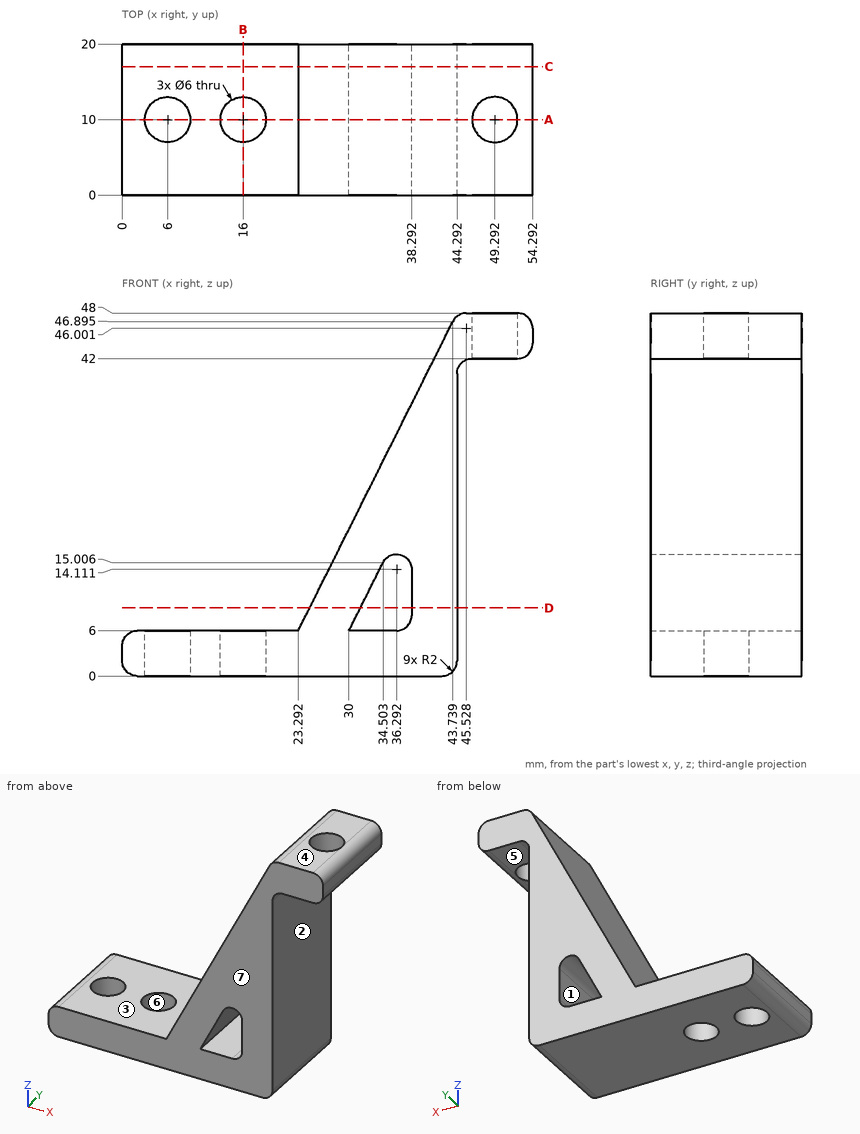
Check sheet for the drawn part. Datum: minimum x, y, z corner. Units: mm. A direction names the side the tool comes from. Round coordinates to 2 decimals unless told otherwise and drop trailing zeros. Loops run counter-clockwise (first coordinate to the right, second up) from the corner with the lowest first, then second, coordinate; pieces in that order, holes last. Notation, with made-up numbers: (80, 10) - (114, 10) arc R13 cw to (114, 29) - close; hole circle Ø8 at (8.25, -23.5). An arc over 180 degrees is marked (long way). Write item = value, one per line. Start each with the question number.
1. Section check D-D on z = 9. Enter the section's corners in (x, y).
2. Depth check by flat-ended pin: pin 1 (5 mm diameter, centred on y = 15, z = 16.5, fed in from -X); pin 2 (3 mm diameter, centred on x = 19.5, y = 10.5, fed in from +Z); pin 3 (7 mm diameter, centred on x = 32.5, y = 10, fed in from +Z) (1 decimal). Enter the tip coordinate at first touch or a pass-through.
3. Set-up check for the marked faces 1, 2, 3 and 4: record each of +Z, -Z, +X, -X, +Y, -Y from which the full face is reachable in a straight line by a thin tool's end or side.
4. Section check C-C on y = 17. Enter the section's corners in (x, z) (1 decimal), then the cut area to 3 significant figures.
5. Thickness scan on line 1 (Y direction, x = 6, z = 2.9); line 2 (X direction, y = 8.75, z = 12.5); line 3 (Z direction, x = 18, y = 7.5). Record the ranges inside material, lowest first.
6. Section check B-B on x = 16. Enter the section's corners in (y, z).
7. Section check A-A on y = 10. Give the number of separate pieces and of enclosed holes in the cut face, then the cut area to 3 significant figures.
8. Mould release check, pull along Y, two halves, no side actions. Record for the marked faces 5, 6 and 7: released by +Y, released by -Y, zero draft, split by the parting line, or undercut.
Working result:
q1.outline = (24.79, 0) - (31.5, 0) - (31.5, 20) - (24.79, 20) - close; (38.29, 0) - (44.29, 0) - (44.29, 20) - (38.29, 20) - close
q2.pin_1 = 27.29
q2.pin_2 = 6
q2.pin_3 = 31.4
q3.face_1 = +Y, -Y
q3.face_2 = -Z, +X, +Y, -Y
q3.face_3 = +Z, -X, +Y, -Y
q3.face_4 = +Z, +X, -X, +Y, -Y
q4.outline = (0, 2) arc R2 ccw to (2, 0) - (42.3, 0) arc R2 ccw to (44.3, 2) - (44.3, 40) arc R2 cw to (46.3, 42) - (52.3, 42) arc R2 ccw to (54.3, 44) - (54.3, 46) arc R2 ccw to (52.3, 48) - (45.5, 48) arc R2 ccw to (43.7, 46.9) - (23.3, 6) - (2, 6) arc R2 ccw to (0, 4) - close; hole (30, 6) - (36.3, 6) arc R2 ccw to (38.3, 8) - (38.3, 14.1) arc R2 ccw to (34.5, 15) - close
q4.area = 707 mm^2
q5.line_1 = 0 to 7, 13 to 20
q5.line_2 = 26.54 to 33.25, 38.29 to 44.29
q5.line_3 = 0 to 6
q6.outline = (0, 0) - (7, 0) - (7, 6) - (0, 6) - close; (13, 0) - (20, 0) - (20, 6) - (13, 6) - close
q7.separate_pieces = 4
q7.enclosed_holes = 1
q7.area = 599 mm^2
q8.face_5 = zero draft
q8.face_6 = undercut
q8.face_7 = released by -Y
